from build123d import *

# Parameters (mm, degrees)
BOSS_EXTRUDE1_DEPTH = 3
SKETCH3_W           = 147.5
SKETCH3_H           = 3.5
SKETCH3_W_2         = 147
SKETCH3_H_2         = 3
CUT_EXTRUDE2_DEPTH  = 3


with BuildPart() as part:
    # Sketch1 → Boss-Extrude1 (new body)
    with BuildSketch(Plane.XY):
        Polygon((79.894045329, 76.229765013), (148.894045329, 76.229765013), (148.894045329, -58.770234987), (79.894045329, -58.770234987), (-67.167101828, -58.770234987), (-72.167101828, -58.770234987), (-98.167101828, -58.770234987), (-101.167101828, -58.770234987), (-101.167101828, 76.229765013), (-98.167101828, 76.229765013), (-72.167101828, 76.229765013), (-67.167101828, 76.229765013), align=None)
    extrude(amount=-BOSS_EXTRUDE1_DEPTH)

    # Sketch3 → Cut-Extrude2 (cut)
    # profile 1 of 4: a face of its own
    with BuildSketch(Plane.XY):
        with Locations((6.332898172, 56.729765013)):
            Rectangle(SKETCH3_W, SKETCH3_H)
        with Locations((6.332898172, 56.729765013)):
            Rectangle(SKETCH3_W_2, SKETCH3_H_2, mode=Mode.SUBTRACT)
    # profile 2 of 4: a face of its own
    with BuildSketch(Plane.XY):
        with Locations((6.332898172, 25.729765013)):
            Rectangle(SKETCH3_W, SKETCH3_H)
        with Locations((6.332898172, 25.729765013)):
            Rectangle(SKETCH3_W_2, SKETCH3_H_2, mode=Mode.SUBTRACT)
    # profile 3 of 4: a face of its own
    with BuildSketch(Plane.XY):
        with Locations((6.332898172, -5.270234987)):
            Rectangle(SKETCH3_W, SKETCH3_H)
        with Locations((6.332898172, -5.270234987)):
            Rectangle(SKETCH3_W_2, SKETCH3_H_2, mode=Mode.SUBTRACT)
    # profile 4 of 4: a face of its own
    with BuildSketch(Plane.XY):
        with Locations((6.332898172, -36.270234987)):
            Rectangle(SKETCH3_W, SKETCH3_H)
        with Locations((6.332898172, -36.270234987)):
            Rectangle(SKETCH3_W_2, SKETCH3_H_2, mode=Mode.SUBTRACT)
    extrude(amount=-CUT_EXTRUDE2_DEPTH, mode=Mode.SUBTRACT)


with BuildPart() as body_2:
    # of the pieces the cut leaves, the one that is kept (cut_extrude2_keep)
    add(part.part.solids().sort_by_distance((148.894045329, 76.229765013, 0))[0])


solid = body_2.part
Here's how the part is built. I have some questions about the finished solid (model axes, mm). Round coordinates to 2 decimals unless told otherwise and drop trailing zeros. Order: outer loops, then holes, each group sorted by start corner. A loop starts at its lowest first (then second) coordinate and runs counter-clockwise, first axis right, second up. Notation, with made-up numbers: (0, 78.25) -> (35, 78.25) arc R32 ccw to (35, 106.25) -> close; hole circle Ø9 at (0.25, 86.5). An arc over 180 degrees is marked (long way). Return JSON: item names as keys, results as strings.
Q1. If we section it at B-B on z = -1.3: List the corners of the cut face in (x, y) for me, plus the area to 3 significant figures.
Filled sheet:
{"outline": "(-101.17, -58.77) -> (148.89, -58.77) -> (148.89, 76.23) -> (-101.17, 76.23) -> close; hole (-67.42, -38.02) -> (80.08, -38.02) -> (80.08, -34.52) -> (-67.42, -34.52) -> close; hole (-67.42, -7.02) -> (80.08, -7.02) -> (80.08, -3.52) -> (-67.42, -3.52) -> close; hole (-67.42, 23.98) -> (80.08, 23.98) -> (80.08, 27.48) -> (-67.42, 27.48) -> close; hole (-67.42, 54.98) -> (80.08, 54.98) -> (80.08, 58.48) -> (-67.42, 58.48) -> close", "area": "31,700 mm^2"}
Q2. If we section it at A-A on x = -59.5: List the corners of the cut face in (y, z) for me.
Filled sheet:
{"outline": "(-58.77, -3) -> (-38.02, -3) -> (-38.02, 0) -> (-58.77, 0) -> close; (-34.52, -3) -> (-7.02, -3) -> (-7.02, 0) -> (-34.52, 0) -> close; (-3.52, -3) -> (23.98, -3) -> (23.98, 0) -> (-3.52, 0) -> close; (27.48, -3) -> (54.98, -3) -> (54.98, 0) -> (27.48, 0) -> close; (58.48, -3) -> (76.23, -3) -> (76.23, 0) -> (58.48, 0) -> close"}
Q3. I need wall thicknesses on line 1 along Y through (x, z) = (75, -1.8); line 2 along X through (y, z) = (-35, -1). Which ranges of each line are inside material? Lowest first, please. Write a range as from..to.
Filled sheet:
{"line 1": "y = -58.77..-38.02, -34.52..-7.02, -3.52..23.98, 27.48..54.98, 58.48..76.23", "line 2": "x = -101.17..-67.42, 80.08..148.89"}
